Design review of the part built by this model. Coordinates are the model's own, in mm. A direction names the side the tool comes from. Give positions to 0.01 mm unless a question says otherwise; leave off trailing zeros. Answer as CSV lines item,"result".
Autodesk Inventor part; units mm, degrees
ref_plane "YZ Plane" through (0, 0, 0) normal (1, 0, 0) x (0, 1, 0)
ref_plane "XZ Plane" through (0, 0, 0) normal (0, 1, 0) x (-1, 0, 0)
ref_plane "XY Plane" through (0, 0, 0) normal (0, 0, 1) x (1, 0, 0)
sketch "Sketch1" plane through (0, 0, 0) normal (0, 0, 1) x (1, 0, 0)
  line L0 (50, -20) -> (8, -20)
  line L1 (8, -17) -> (50, -17)
  line L2 (50, -17) -> (50, -20)
  line L3 (8, -20) -> (8, -17)
  line L4 (50, -17) -> (8, -17)
  line L5 (8, -17) -> (8, -20)
  line L6 (8, -20) -> (50, -20)
  line L7 (50, -20) -> (50, -17)
  point P0 (0, 0)
extrude "Extrusion1" add sketch "Sketch1" along normal blind 76
sketch "Sketch2" plane through (50, -20, 0) normal (1, 0, 0) x (0, 0, -1)
  line L0 (-73, 6.5) -> (-73, 16.5)
  line L1 (0, 3) -> (-76, 3)
  line L2 (0, 0) -> (0, 3)
  line L3 (0, 0) -> (-76, 0)
  line L4 (-73, 0) -> (0, 0)
  line L5 (0, 0) -> (0, 3)
  line L6 (0, 3) -> (-73, 3)
  line L7 (-73, 3) -> (-73, 0)
  point P0 (0, 20)
  point P1 (-69, 3)
  point P2 (-69, 1.5)
  point P3 (-73, 3)
extrude "Extrusion2" add sketch "Sketch2" along normal blind 10
sketch "Sketch3" plane through (8, -20, 0) normal (-1, 0, 0) x (0, 0, 1)
  line L0 (73, 6.5) -> (73, 16.5)
  line L1 (0, 3) -> (0, 0)
  line L2 (0, 3) -> (76, 3)
  line L3 (73, 3) -> (0, 3)
  line L4 (0, 3) -> (0, 0)
  line L5 (0, 0) -> (73, 0)
  line L6 (73, 0) -> (73, 3)
  point P0 (0, 20)
  point P1 (69, 0)
  point P2 (69, 1.5)
extrude "Extrusion3" add sketch "Sketch3" along normal blind 10
properties part number "divider 2"
Q1. For faces 1 (the flat face through (55, -18, 73)), 2 (the flat face through (29, -20, 37)), 3 (the flat face through (8, -19, 74)), list the 3-axis set-ups (+Z, -Z, +X, -X, +Y, -Y) from which the entire face can be reached by the end or side of a thin tool; tool diameter is ignored.
Filled sheet:
face 1,"+Z, +X, +Y, -Y"
face 2,"+Z, -Z, +X, -X, -Y"
face 3,"+Z, -X, +Y, -Y"
Q2. To check wall thickness, follow probe 1 along Z at (x, y) = (1, -18.25). State the ranges of the line that lie inside material, in increasing order. Write a range as from..to.
Filled sheet:
probe 1,"z = 0..73"
Q3. Clearance check with flat-ended pins moving along their axes: pin 1 Ø0.9 at (y, z) = (-18.5, 74) entering from -X; pin 2 Ø1.5 at (x, y) = (2.5, -19) entering from +Z; pin 3 Ø0.9 at (y, z) = (-18, 74) entering from +X. State where each tip first meets the part, or that it passes through.
Filled sheet:
pin 1,"stops at x = 8"
pin 2,"stops at z = 73"
pin 3,"stops at x = 50"
